Design review of the part built by this model. Coordinates are the model's own, in mm. A direction names the side the tool comes from. Coordinates: 2 decimals unless noted, no trailing zeros. Order: outer loops, then holes, each group sorted by start corner. A loop starts at its lowest first (then second) coordinate and runs counter-clockwise, first axis right, second up. Notation, with made-up numbers: M 61.5,-6 L 106.5,-6 A15 ccw 106.5,20 Z; hole C -12,-17.5 d6. An arc over 180 degrees is marked long. Answer as a JSON object with one key per item and string values.
from build123d import *

# Parameters (mm, degrees)
SKETCH1_R               = 9.525
BOSS_EXTRUDE1_DEPTH     = 38.1
SKETCH2_R               = 12.7
BOSS_EXTRUDE2_DEPTH     = 12.7
SKETCH3_R               = 9.525
BOSS_EXTRUDE3_DEPTH     = 76.2
SKETCH4_R               = 10.795
BOSS_EXTRUDE4_DEPTH     = 19.05
BOSS_EXTRUDE5_DEPTH     = 10.16
SKETCH6_R               = 8.255
BOSS_EXTRUDE6_DEPTH     = 5.08
SKETCH7_R               = 3.175
BOSS_EXTRUDE7_DEPTH     = 22.86
CUT_EXTRUDE1_DEPTH      = 22.86
CUT_EXTRUDE1_DEPTH_BACK = 22.86
SKETCH8_R               = 5.08
SKETCH9_W               = 16.087027097
SKETCH9_H               = 5.943828254
CUT_EXTRUDE2_DEPTH      = 38.1


with BuildPart() as part:
    # Sketch1 → Boss-Extrude1 (new body)
    with BuildSketch(Plane.XY):
        with Locations(Location((0, 0, 0), (0, 0, 180))):
            Circle(SKETCH1_R)
    extrude(amount=BOSS_EXTRUDE1_DEPTH)

    # Sketch2 → Boss-Extrude2 (add)
    with BuildSketch(Plane.XY.offset(38.1)):
        Circle(SKETCH2_R)
    extrude(amount=BOSS_EXTRUDE2_DEPTH)

    # Sketch3 → Boss-Extrude3 (add)
    with BuildSketch(Plane.XY.offset(50.8)):
        with Locations(Location((0, 0, 0), (0, 0, 180))):
            Circle(SKETCH3_R)
    extrude(amount=BOSS_EXTRUDE3_DEPTH)

    # Sketch4 → Boss-Extrude4 (add)
    with BuildSketch(Plane.XY.offset(127)):
        with Locations(Location((0, 0, 0), (0, 0, 180))):
            Circle(SKETCH4_R)
    extrude(amount=BOSS_EXTRUDE4_DEPTH)

    # Sketch5 → Boss-Extrude5 (add)
    with BuildSketch(Plane.XY.offset(146.05)):
        Polygon((-7.663715272, 13.97), (7.663715272, 13.97), (13.97, 0), (7.663715272, -13.97), (-7.663715272, -13.97), (-13.97, 0), align=None)
    extrude(amount=BOSS_EXTRUDE5_DEPTH)

    # Sketch6 → Boss-Extrude6 (add)
    with BuildSketch(Plane.XY.offset(156.21)):
        with Locations(Location((0, 0, 0), (0, 0, 180))):
            Circle(SKETCH6_R)
    extrude(amount=BOSS_EXTRUDE6_DEPTH)

    # Sketch7 → Boss-Extrude7 (add)
    with BuildSketch(Plane.XY.offset(161.29)):
        Circle(SKETCH7_R)
    extrude(amount=BOSS_EXTRUDE7_DEPTH)

    # Sketch8 → Cut-Extrude1 (cut, two sides: drawn at the far end of the back side and taken through both)
    with BuildSketch(Plane(origin=(0, 0, 0), x_dir=(1, 0, 0), z_dir=(0, 1, 0)).offset(-CUT_EXTRUDE1_DEPTH_BACK)):
        with Locations(Location((0, -25.4, 0), (0, 0, 90))):
            Circle(SKETCH8_R)
    extrude(amount=CUT_EXTRUDE1_DEPTH + CUT_EXTRUDE1_DEPTH_BACK, mode=Mode.SUBTRACT)

    # Sketch9 → Cut-Extrude2 (cut)
    with BuildSketch(Plane(origin=(0, 0, 0), x_dir=(-1, 0, 0), z_dir=(0, 0, -1))):
        with Locations((1.010043222, 9.394991284)):
            Rectangle(SKETCH9_W, SKETCH9_H)
    cut_extrude2 = extrude(amount=-CUT_EXTRUDE2_DEPTH, mode=Mode.SUBTRACT)

    # Mirror1: Cut-Extrude2 across plane
    add(cut_extrude2.mirror(Plane.ZX), mode=Mode.SUBTRACT)


solid = part.part
1) Add section A-A (z = 25.4). State the section outline as (x, y) points (3 decimals).
Taken from the geometry:
{"outline": "M -7.033,-6.423 L -5.08,-6.423 L -5.08,6.423 L -7.033,6.423 A9.525 ccw Z; M 5.08,-6.423 L 7.033,-6.423 A9.525 ccw 7.033,6.423 L 5.08,6.423 Z"}
2) Add section C-C (z = 143.5). State the section outline as (x, y) points (3 decimals).
Taken from the geometry:
{"outline": "C 0,0 d21.59"}
3) Tool access review of faces 1 (the cylindrical face through (-9.524, 0.099, 18.783)), 2 (the flat face through (0, 10, 127)), 3 (the flat face through (0, -6.423, 19)), 4 (the cylindrical face through (9.524, -0.099, 18.783)): name each direction out of +Z, -Z, +X, -X, +Y, -Y from which nothing blocks a thin tool from reaching the whole face with its end or side.
Taken from the geometry:
{"face 1": "-Z, -X", "face 2": "none", "face 3": "-Z, +X, -X, -Y", "face 4": "-Z, +X"}
4) Insertion check: pin 1 Ø8.5 at (x, y) = (-6.5, 5.5) entering from +Z; pin 2 Ø3 at (x, z) = (-4.5, 23.5) entering from -Y; pin 3 Ø1.5 at (x, z) = (-9, 129.5) entering from -Y; pin 4 Ø4 at (x, z) = (-2.5, 25) entering from -Y. Each pin has a flat end and moves straight along its axis. Give the tip position at first contact, or say it passes through.
Taken from the geometry:
{"pin 1": "stops at z = 161.29", "pin 2": "stops at y = -6.42", "pin 3": "stops at y = -6.96", "pin 4": "passes through"}
5) To check wall thickness, follow L1, parallel to Z at x = 1.25, y = -10.5; L2, parallel to X at y = 3.25, z = 25.4; L3, parallel to Z at x = -0.5, y = 5.25. State the ranges of each line that lie inside material, in increasing order.
Taken from the geometry:
{"L1": "z = 38.1 to 50.8, 127 to 156.21", "L2": "x = -8.95 to -5.08, 5.08 to 8.95", "L3": "z = 0 to 20.34, 30.46 to 161.29"}
6) Add section D-D (z = 166.5). State the section outline as (x, y) points (3 decimals).
Taken from the geometry:
{"outline": "C 0,0 d6.35"}
7) Mouldability with a two-part tool opening along Z and no side actions: class faces 5 (the flat face through (0, 4, 161.29)), 6 (the flat face through (7.3, -8.2, 146.05)), 7 (the flat face through (0, 6.423, 19)), 8 (the flat face through (0, -8, 38.1)) as released by +Z, released by -Z, zero draft, split by the parting line, or undercut.
Taken from the geometry:
{"face 5": "released by +Z", "face 6": "undercut", "face 7": "zero draft", "face 8": "released by -Z"}
